For this review, take the finished solid that the model builds, in its own axes (mm). A direction names the side the tool comes from. Give positions to 0.01 mm unless a question says otherwise; leave off trailing zeros. Order: outer loops, then holes, each group sorted by start corner. A loop starts at its lowest first (then second) coordinate and runs counter-clockwise, first axis right, second up. Notation, with made-up numbers: (74, -25) -> (99, -25) arc R25 cw to (99, -3) -> close; hole circle Ø7 at (-1, -31.75). An arc over 180 degrees is marked (long way). One line per item, written item: value. Start each with the question number.
from build123d import *

# Parameters (mm, degrees)
BOSS_EXTRUDE1_DEPTH = 1.27
CUT_EXTRUDE2_DEPTH  = 64.13835029
SKETCH4_R           = 1.27
SKETCH4_R_2         = 1.5875
CUT_EXTRUDE3_DEPTH  = 64.13835029


with BuildPart() as part:
    # Sketch1 → Boss-Extrude1 (new body)
    with BuildSketch(Plane.XY):
        with BuildLine():
            Line((-6.832612328, -62.148292065), (6.8326, -62.148292065))
            ThreePointArc((6.8326, -62.148292065), (9.145004667, -61.82662212), (10.217979737, -59.753119914))
            Line((10.217979737, -59.753119914), (10.217979737, -50.431712328))
            Line((10.217979737, -50.431712328), (6.839792065, -29.750592065))
            Line((6.839792065, -29.750592065), (2.667806008, -0.146870092))
            ThreePointArc((2.667806008, -0.146870092), (2.653236727, -0.020752709), (2.644987367, 0.105935121))
            ThreePointArc((2.644987367, 0.105935121), (1.833951843, 1.908874292), (0, 2.647107935))
            add(Edge.make_bspline(
                [(0, 2.647107935), (-0.561984482, 2.60663561), (-0.837703259, 2.51106226)],
                knots=[0, 0, 0, 0.00724911, 0.00724911, 0.00724911], degree=2))
            ThreePointArc((-0.837703259, 2.51106226), (-1.617455697, 2.09547548), (-2.216994409, 1.446414952))
            add(Edge.make_bspline(
                [(-2.216994409, 1.446414952), (-2.348446751, 1.249612458), (-2.562206256, 0.722759125), (-2.600800514, 0.492967657)],
                knots=[0.022131974, 0.022131974, 0.022131974, 0.022131974, 0.030911059, 0.030911059, 0.030911059, 0.030911059], degree=3))
            ThreePointArc((-2.600800514, 0.492967657), (-2.63362686, 0.266814516), (-2.646825425, 0.038672871))
            ThreePointArc((-2.646825425, 0.038672871), (-2.647287537, 0.01475577), (-2.647974875, -0.009155919))
            add(Edge.make_bspline(
                [(-2.647974875, -0.009155919), (-2.982966974, -10.021345785), (-5.211696232, -26.748717576), (-8.559038061, -43.581295567), (-9.3726, -50.4317)],
                knots=[0.035874882, 0.035874882, 0.035874882, 0.035874882, 0.412185068, 0.675162616, 0.675162616, 0.675162616, 0.675162616], degree=3))
            Line((-9.3726, -50.4317), (-9.3726, -59.608304393))
            ThreePointArc((-9.3726, -59.608304393), (-8.628654835, -61.4043469), (-6.832612328, -62.148292065))
        make_face()
    extrude(amount=BOSS_EXTRUDE1_DEPTH)

    # Sketch2 → Cut-Extrude2 (cut, through all)
    with BuildSketch(Plane.XY.offset(1.27)):
        with BuildLine():
            ThreePointArc((1.5875, -62.148292065), (0, -60.560792065), (-1.5875, -62.148292065))
            Line((-1.5875, -62.148292065), (1.5875, -62.148292065))
        make_face()
        with BuildLine():
            Line((-2.993002621, -52.629071042), (2.993002621, -52.629071042))
            ThreePointArc((2.993002621, -52.629071042), (3.726800948, -52.31577725), (4.008051125, -51.569110442))
            add(Edge.make_bspline(
                [(4.008051125, -51.569110442), (3.970454208, -50.700999098), (3.762157848, -48.039220625), (3.064677271, -43.892588352), (2.039593657, -39.517305496), (1.382803309, -36.905376029), (1.10391193, -35.774249306)],
                knots=[0.059039804, 0.059039804, 0.059039804, 0.059039804, 0.20424764, 0.505314101, 0.760840146, 0.955648589, 0.955648589, 0.955648589, 0.955648589], degree=3))
            ThreePointArc((1.10391193, -35.774249306), (0.744009182, -35.217668165), (0.11745403, -35.001471042))
            Line((0.11745403, -35.001471042), (-0.11745403, -35.001471042))
            ThreePointArc((-0.11745403, -35.001471042), (-0.744009182, -35.217668165), (-1.10391193, -35.774249306))
            add(Edge.make_bspline(
                [(-4.008051125, -51.569110442), (-3.970454208, -50.700999098), (-3.762157848, -48.039220625), (-3.064677271, -43.892588352), (-2.039593657, -39.517305496), (-1.382803309, -36.905376029), (-1.10391193, -35.774249306)],
                knots=[0.059039804, 0.059039804, 0.059039804, 0.059039804, 0.20424764, 0.505314101, 0.760840146, 0.955648589, 0.955648589, 0.955648589, 0.955648589], degree=3))
            ThreePointArc((-4.008051125, -51.569110442), (-3.726800948, -52.31577725), (-2.993002621, -52.629071042))
        make_face()
    extrude(amount=-CUT_EXTRUDE2_DEPTH, mode=Mode.SUBTRACT)

    # Sketch4 → Cut-Extrude3 (cut, through all)
    with BuildSketch(Plane(origin=(0, 0, 0), x_dir=(-1, 0, 0), z_dir=(0, 0, -1))):
        with Locations((4.407451174, -57.57698217)):
            Circle(SKETCH4_R)
        with Locations((-4.571309894, -57.740840891)):
            Circle(SKETCH4_R)
        with Locations((0.210042576, 0.287306268)):
            Circle(SKETCH4_R_2)
    extrude(amount=-CUT_EXTRUDE3_DEPTH, mode=Mode.SUBTRACT)


solid = part.part
Q1. For pin 1 Ø0.6 at (x, z) = (-4, 0.5) entering from -Y, flat-tipped, find the tip position at first contact; note if it passes through.
Q2. For line 1 along Y through (x, z) = (-1, 1.2); line 2 along X through (y, z) = (-57, 0.5); line 3 along X through (y, z) = (-51.5, 0.45) (3 decimals), list the stretches that pass through material, from the lowest coordinate up.
Q3. Mouldability with a two-part tool opening along Y and no side actions: class faces 1 (the cylindrical face through (-1.724, 0.764, 0.626)), 2 (the flat face through (2, -37, 1.27)), 3 (the flat face through (-4, -62.148, 1)) as pulls with the +Y half, pulls with the -Y half, needs draft (parallel to the pull), parting line crosses it, or undercut.
Q4. Take a section at B-B (x = 7.75). State the section outline as (y, z) points, and give its area (3 significant figures).
Q5. Take a section at A-A (z = 0.6). State how many separate pieces and enclosed holes the cut face has, and give its area (3 significant figures).
Q6. For faces 4 (the cylindrical face through (1.854, 1.889, 0.626)), 5 (the flat face through (4, -62.148, 1)), 6 (the cylindrical face through (-3.73, -52.31, 0.64)), list the 3-axis set-ups (+Z, -Z, +X, -X, +Y, -Y) from which the entire face can be reached by the end or side of a thin tool; tool diameter is ignored.
Answers below:
1. pin 1: stops at y = -62.15
2. line 1: y = -60.92 to -52.63, -35.51 to -1.09, 1.66 to 2.45
2. line 2: x = -9.37 to -5.54, -3.28 to 3.54, 5.6 to 10.22
2. line 3: x = -9.373 to -4.005, 4.005 to 10.218
3. face 1: undercut
3. face 2: needs draft
3. face 3: pulls with the -Y half
4. outline: (-62.29, 0) -> (-35.32, 0) -> (-35.32, 1.27) -> (-62.29, 1.27) -> close
4. area: 34.3 mm²
5. separate pieces: 1
5. enclosed holes: 4
5. area: 714 mm²
6. face 4: +Z, -Z, +X, +Y
6. face 5: +Z, -Z, -X, -Y
6. face 6: +Z, -Z
